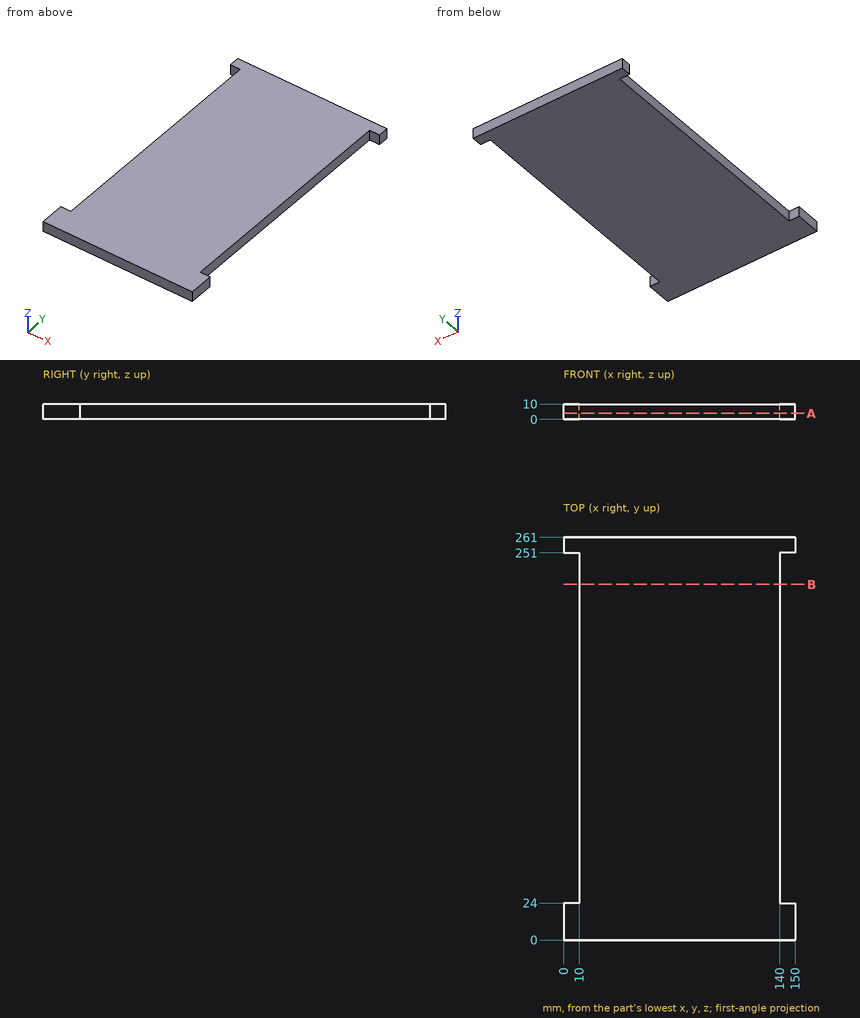
Could you check a few things on this drawing? It's one solid part, dimensions in mm from its lowest x, y, z. Give positions to 0.01 mm unless a question says otherwise; leave off trailing zeros. Order: outer loops, then holes, each group sorted by start corner. A loop starts at its lowest first (then second) coordinate and runs counter-clockwise, first axis right, second up. Notation, with made-up numbers: (8.25, 34.5) - (64.25, 34.5) arc R12 cw to (64.25, 52.5) - close; hole circle Ø1 at (33, 2). An arc over 180 degrees is marked (long way). One line per question, with ' | ' between items. Start each with the question number.
Item 1: I want a section at A-A on z = 4. Write out the boundary of the cut face in (x, y), then the cut area to 3 significant figures.
Item 2: I need wall thicknesses on probe 1 along X at (y, z) = (154, 2); probe 2 along Y at (x, z) = (142, 1). Which ranges of each line are inside material? Lowest first, please. Write a range as [from, to].
Item 3: I'm going to push a flat-ended pin straight in: pin 1 Ø8 at (x, y) = (76.5, 99) entering from -Z. Where does the tip first touch, or does it pass through?
Item 4: I want a section at B-B on y = 230.5. Write out the boundary of the cut face in (x, z), then the cut area to 3 significant figures.
Verdict:
1) outline: (0, 0) - (150, 0) - (150, 24) - (140, 24) - (140, 251) - (150, 251) - (150, 261) - (0, 261) - (0, 251) - (10, 251) - (10, 24) - (0, 24) - close | area: 34,600 mm^2
2) probe 1: [10, 140] | probe 2: [0, 24], [251, 261]
3) pin 1: z = 0
4) outline: (10, 0) - (140, 0) - (140, 10) - (10, 10) - close | area: 1,300 mm^2
